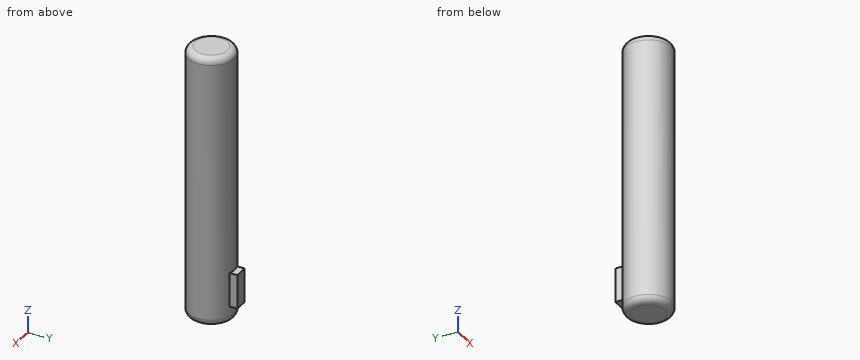
from build123d import *

# Parameters (mm, degrees)
SKETCH1_R           = 3.4
BOSS_EXTRUDE1_DEPTH = 40
FILLET2_R           = 1
BOSS_EXTRUDE2_DEPTH = 5


with BuildPart() as part:
    # Sketch1 → Boss-Extrude1 (new body)
    with BuildSketch(Plane.XY):
        Circle(SKETCH1_R)
    extrude(amount=BOSS_EXTRUDE1_DEPTH)

    # Fillet2
    fillet2_edges = [part.edges().sort_by_distance(p)[0] for p in [
        (-3.4, 0, 0),
        (-3.4, 0, 40),
    ]]
    fillet(fillet2_edges, radius=FILLET2_R)

    # Sketch2 → Boss-Extrude2 (add)
    with BuildSketch(Plane.XY.offset(2.5)):
        with BuildLine():
            Line((1, 3.249615362), (1, 4.399615362))
            Line((1, 4.399615362), (-1, 4.399615362))
            Line((-1, 4.399615362), (-1, 3.249615362))
            ThreePointArc((-1, 3.249615362), (0, 3.4), (1, 3.249615362))
        make_face()
    extrude(amount=BOSS_EXTRUDE2_DEPTH)


solid = part.part
Geometry check sheet. Reference: the model listing, model coordinates, mm. Round coordinates to 2 decimals unless told otherwise and drop trailing zeros. Write each loop counter-clockwise with the first axis right and the second up, starting at its lowest first coordinate (ties: lowest second). Pieces come first, ordered by that corner, then holes. Notation, with made-up numbers: (35.25, -11.75) - (75.25, -11.75) arc R5 ccw to (75.25, -2.75) - close; hole circle Ø9 at (4, 86.25). An arc over 180 degrees is marked (long way). One line per item, written item: value.
1. Cross-section at C-C on z = 27. Record the boundary of the cut face in (x, y).
The answers:
outline: circle Ø6.8 at (0, 0)
2. Cross-section at B-B on z = 4.5. Record the boundary of the cut face in (x, y), and give its area (3 significant figures).
The answers:
outline: (-1, 3.25) arc R3.4 ccw (long way) to (1, 3.25) - (1, 4.4) - (-1, 4.4) - close
area: 38.4 mm^2
3. Scan lines: L1, parallel to Z at x = 0.75, y = 3.5; L2, parallel to X at y = 2.5, z = 22; L3, parallel to X at y = -0.75, z = 6. Record each from-to range of solid material in increasing order.
The answers:
L1: z = 2.5 to 7.5
L2: x = -2.3 to 2.3
L3: x = -3.32 to 3.32
4. Depth check by flat-ended pin: pin 1 Ø0.9 at (y, z) = (4, 4.5) entering from +X; pin 2 Ø1 at (x, z) = (-1, 11.5) entering from +Y; pin 3 Ø1.3 at (x, y) = (0, 3.5) entering from +Z. Enter the tip coordinate at first touch or a pass-through.
The answers:
pin 1: stops at x = 1
pin 2: stops at y = 3.36
pin 3: stops at z = 39.89
5. Cross-section at A-A on x = 0. Record the boundary of the cut face in (y, z).
The answers:
outline: (-3.4, 1) arc R1 ccw to (-2.4, 0) - (2.4, 0) arc R1 ccw to (3.4, 1) - (3.4, 2.5) - (4.4, 2.5) - (4.4, 7.5) - (3.4, 7.5) - (3.4, 39) arc R1 ccw to (2.4, 40) - (-2.4, 40) arc R1 ccw to (-3.4, 39) - close
